from build123d import *

# Parameters (mm, degrees)
BOSS_EXTRUDE1_DEPTH    = 457.2
CONVERT_SOLID1_DEPTH   = 457.2
CONVERT_SOLID1_2_DEPTH = 457.2


# Read off the part's stored shape, not the designer's step: Convert-Solid1
with BuildPart() as part:
    # Sketch1 → Boss-Extrude1 (new body)
    with BuildSketch(Plane(origin=(0, 0, 0), x_dir=(0, 0, 1), z_dir=(1, 0, 0))):
        Polygon((-29.751953414, 596.435252585), (-65.16880823, 409.640335681), (-63.546707453, 409.332780696), (-28.059593886, 596.498254998), (-28.279614725, 597.319383946), (-44.285546712, 657.054335345), (-44.538099225, 657.996874156), (-45.228085523, 658.686860454), (-88.95625047, 702.415025401), (-89.646236768, 703.105011699), (-90.588775579, 703.357564213), (-150.322559758, 719.363183444), (-151.265098569, 719.615735957), (-152.20763738, 719.363183444), (-211.941421559, 703.357564213), (-212.88396037, 703.105011699), (-213.573946668, 702.415025401), (-257.302111615, 658.686860454), (-257.992097913, 657.996874156), (-258.244650426, 657.054335345), (-274.250582413, 597.319383946), (-274.470603252, 596.498254998), (-238.983489685, 409.332780696), (-237.361388908, 409.640335681), (-272.778243724, 596.435252585), (-272.655838874, 596.892073703), (-256.649906887, 656.627025102), (-256.511851808, 657.14225367), (-256.134678319, 657.519427159), (-212.406513372, 701.247592106), (-212.029339883, 701.624765595), (-211.514111315, 701.762820673), (-151.780327137, 717.768439905), (-151.265098569, 717.906494983), (-150.749870001, 717.768439905), (-91.016085823, 701.762820673), (-90.500857255, 701.624765595), (-90.123683766, 701.247592106), (-46.395518819, 657.519427159), (-46.01834533, 657.14225367), (-45.880290251, 656.627025102), (-29.874358264, 596.892073703), align=None)
    extrude(amount=BOSS_EXTRUDE1_DEPTH)

    # Convert-Solid1 outline → Convert-Solid1 (cut)
    with BuildSketch(Plane.YZ):
        with BuildLine():
            Line((-409.332780696, -238.983489685), (-409.360909589, -238.8351328))
            Line((-409.360909589, -238.8351328), (-595.819160173, -274.188154711))
            ThreePointArc((-595.819160173, -274.188154711), (-596.489617721, -274.238590248), (-597.154469491, -274.138444405))
            Line((-597.154469491, -274.138444405), (-657.14225367, -258.064766079))
            ThreePointArc((-657.14225367, -258.064766079), (-657.865796534, -257.765064811), (-658.487116878, -257.288308944))
            Line((-658.487116878, -257.288308944), (-702.40122273, -213.374203091))
            ThreePointArc((-702.40122273, -213.374203091), (-702.877978598, -212.752882748), (-703.177679865, -212.029339883))
            Line((-703.177679865, -212.029339883), (-719.251358192, -152.041555704))
            ThreePointArc((-719.251358192, -152.041555704), (-719.353580713, -151.265098569), (-719.251358192, -150.488641434))
            Line((-719.251358192, -150.488641434), (-703.177679865, -90.500857255))
            ThreePointArc((-703.177679865, -90.500857255), (-702.877978598, -89.77731439), (-702.40122273, -89.155994047))
            Line((-702.40122273, -89.155994047), (-658.487116878, -45.241888194))
            ThreePointArc((-658.487116878, -45.241888194), (-657.865796534, -44.765132327), (-657.14225367, -44.465431059))
            Line((-657.14225367, -44.465431059), (-597.154469491, -28.391752733))
            ThreePointArc((-597.154469491, -28.391752733), (-596.489617721, -28.29160689), (-595.819160173, -28.342042427))
            Line((-595.819160173, -28.342042427), (-409.360909589, -63.695064338))
            Line((-409.360909589, -63.695064338), (-409.332780696, -63.546707453))
            Line((-409.332780696, -63.546707453), (-596.498254998, -28.059593886))
            Line((-596.498254998, -28.059593886), (-657.996874156, -44.538099225))
            Line((-657.996874156, -44.538099225), (-703.105011699, -89.646236768))
            Line((-703.105011699, -89.646236768), (-719.615735957, -151.265098569))
            Line((-719.615735957, -151.265098569), (-703.105011699, -212.88396037))
            Line((-703.105011699, -212.88396037), (-657.996874156, -257.992097913))
            Line((-657.996874156, -257.992097913), (-596.498254998, -274.470603252))
            Line((-596.498254998, -274.470603252), (-409.332780696, -238.983489685))
        make_face()
    extrude(amount=CONVERT_SOLID1_DEPTH, mode=Mode.SUBTRACT)

    # Convert-Solid1 2 outline → Convert-Solid1 2 (add)
    with BuildSketch(Plane.YZ):
        with BuildLine():
            ThreePointArc((-596.098586265, -272.714410818), (-596.433815038, -272.739628587), (-596.766240923, -272.689555666))
            Line((-596.766240923, -272.689555666), (-596.435252585, -272.778243724))
            Line((-596.435252585, -272.778243724), (-596.098586265, -272.714410818))
        make_face()
        with BuildLine():
            Line((-657.14225367, -256.511851808), (-656.754025102, -256.615877339))
            ThreePointArc((-656.754025102, -256.615877339), (-657.115796534, -256.466026706), (-657.426456706, -256.227648772))
            Line((-657.426456706, -256.227648772), (-657.14225367, -256.511851808))
        make_face()
        with BuildLine():
            Line((-701.624765595, -212.029339883), (-701.340562558, -212.313542919))
            ThreePointArc((-701.340562558, -212.313542919), (-701.578940492, -212.002882747), (-701.728791126, -211.641111315))
            Line((-701.728791126, -211.641111315), (-701.624765595, -212.029339883))
        make_face()
        with BuildLine():
            Line((-717.906494983, -151.265098569), (-717.802469452, -151.653327137))
            ThreePointArc((-717.802469452, -151.653327137), (-717.853580713, -151.265098569), (-717.802469452, -150.876870001))
            Line((-717.802469452, -150.876870001), (-717.906494983, -151.265098569))
        make_face()
        with BuildLine():
            Line((-701.624765595, -90.500857255), (-701.728791126, -90.889085823))
            ThreePointArc((-701.728791126, -90.889085823), (-701.578940492, -90.527314391), (-701.340562558, -90.216654219))
            Line((-701.340562558, -90.216654219), (-701.624765595, -90.500857255))
        make_face()
        with BuildLine():
            Line((-657.14225367, -46.01834533), (-657.426456706, -46.302548366))
            ThreePointArc((-657.426456706, -46.302548366), (-657.115796534, -46.064170432), (-656.754025102, -45.914319799))
            Line((-656.754025102, -45.914319799), (-657.14225367, -46.01834533))
        make_face()
        with BuildLine():
            Line((-596.435252585, -29.751953414), (-596.766240923, -29.840641472))
            ThreePointArc((-596.766240923, -29.840641472), (-596.433815038, -29.790568551), (-596.098586265, -29.815786319))
            Line((-596.098586265, -29.815786319), (-596.435252585, -29.751953414))
        make_face()
    extrude(amount=CONVERT_SOLID1_2_DEPTH)


solid = part.part
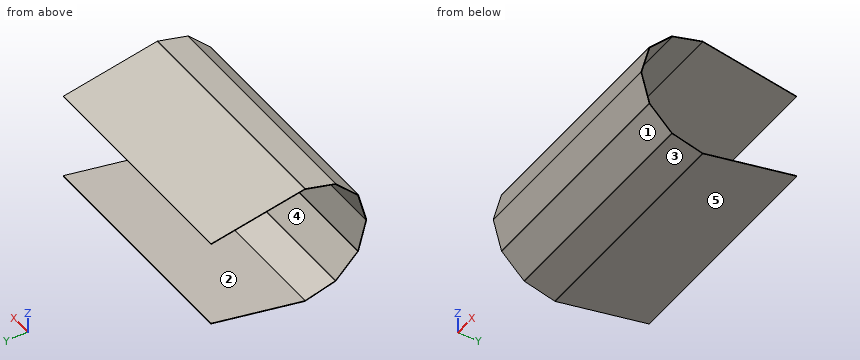
Work out the finished part from the listing and answer in its coordinate system (mm). Face numbers are marked on the shaded views. A direction names the side the tool comes from. Give positions to 0.01 mm unless a question says otherwise; leave off trailing zeros. Loops run counter-clockwise (first coordinate to the right, second up) from the corner with the lowest first, then second, coordinate; pieces in that order, holes last. Notation, with made-up numbers: (18, 3) -> (65, 3) arc R18 cw to (65, 7) -> close; hole circle Ø1 at (18.25, 4.25). An arc over 180 degrees is marked (long way). Use a Markdown table: item, result. Add a question column.
1. Section C-C on z = -132 is taken. Determine the outline of the cut face in (x, y), and give its area (3 significant figures).
2. Find the intervals of material crossed by probe 1 along Z at (x, y) = (260, -597); probe 2 along Z at (x, y) = (390, -619); probe 3 along Y at (x, z) = (39, -151.5), in increasing order.
3. Section B-B on y = -644 is taken. Determine the outline of the cut face in (x, z).
4. Determine the mould class of the marked faces 3, 4 and 5 for opening direction Y: released by +Y, released by -Y, zero draft, split by the parting line, or undercut.
5. For the marked faces 1 and 2, determine the directions among +Z, -Z, +X, -X, +Y, -Y from which every point of the face is accessible in a straight line to the end or side of a thin tool.
6. Flat-ended cylindrical pins translate along their axes: pin 1 Ø2 at (x, y) = (65.5, -569) entering from -Z; pin 2 Ø4 at (x, z) = (161, -207) entering from -Y; pin 3 Ø2 at (x, y) = (53.5, -527.5) entering from -Z; pin 4 Ø10 at (x, y) = (225.5, -592) entering from -Z. Find the tip coordinate at first contact, or state that the pin passes through.
7. Section A-A on z = -246 is taken. Determine the outline of the cut face in (x, y), and give its area (3 significant figures).
Results below:
| question | item | result |
|---|---|---|
| 1 | outline | (0, -714.3) -> (457.2, -714.3) -> (457.2, -712.74) -> (0, -712.74) -> close |
| 1 | area | 710 mm^2 |
| 2 | probe 1 | z = -274.18 to -272.63, -29.9 to -28.35 |
| 2 | probe 2 | z = -268.28 to -266.73, -35.8 to -34.25 |
| 2 | probe 3 | y = -719.34 to -717.84 |
| 3 | outline | (0, -261.59) -> (457.2, -261.59) -> (457.2, -260.03) -> (0, -260.03) -> close; (0, -42.5) -> (457.2, -42.5) -> (457.2, -40.94) -> (0, -40.94) -> close |
| 4 | face 3 | released by -Y |
| 4 | face 4 | undercut |
| 4 | face 5 | released by +Y |
| 5 | face 1 | -Z, +X, -X, -Y |
| 5 | face 2 | +X, -X |
| 6 | pin 1 | stops at z = -269.29 |
| 6 | pin 2 | stops at y = -705.06 |
| 6 | pin 3 | stops at z = -261.42 |
| 6 | pin 4 | stops at z = -274.24 |
| 7 | outline | (0, -669.78) -> (457.2, -669.78) -> (457.2, -667.65) -> (0, -667.65) -> close; (0, -455.2) -> (457.2, -455.2) -> (457.2, -447.15) -> (0, -447.15) -> close |
| 7 | area | 4,650 mm^2 |
